Source: three-view drawing plus pictorial views. Frame: mm from the lowest corner of the part. A direction names the side the tool comes from. Coordinates: 2 decimals unless noted, no trailing zeros. Order: outer loops, then holes, each group sorted by start corner. A loop starts at its lowest first (then second) coordinate and runs counter-clockwise, first axis right, second up. Notation, with made-up numbers: (64.5, -17.75) -> (78.5, -17.75) arc R23 cw to (78.5, 19.25) -> close; hole circle Ø11 at (29.25, -32). An arc over 180 degrees is marked (long way). One line per question, with ' | ' between items.
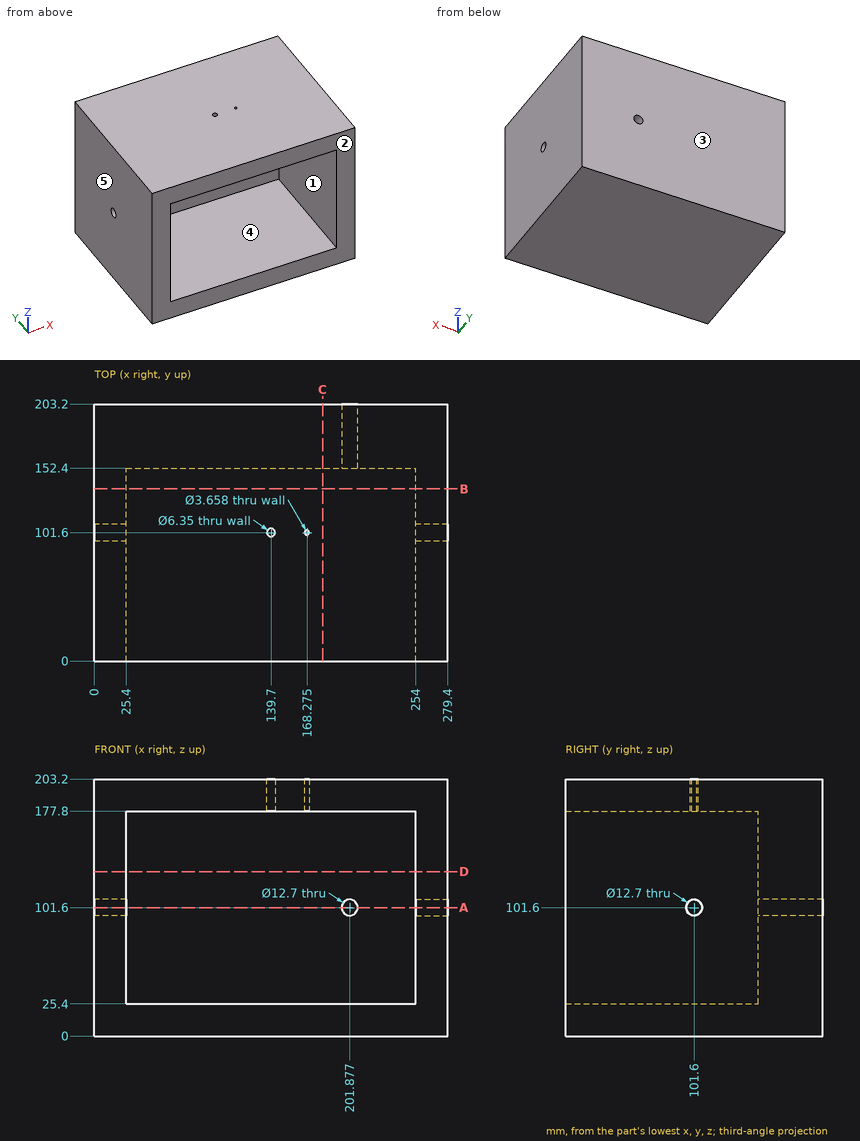
1. Mould query, pull axis X, two halves, no side actions, for the marked faces 3, 4 and 5. Classes: released by +X, released by -X, zero draft, split by the parting line, or undercut.
Recorded:
face 3: zero draft | face 4: undercut | face 5: released by -X
2. Cut plane D-D, the plane z = 130. Return loops of the section in (x, y), and give its area (3 significant figures).
Recorded:
outline: (0, 0) -> (25.4, 0) -> (25.4, 152.4) -> (254, 152.4) -> (254, 0) -> (279.4, 0) -> (279.4, 203.2) -> (0, 203.2) -> close | area: 21,900 mm^2
3. Ray query, line 1 (Z direction, x = 273, y = 101); line 2 (Z direction, x = 197.5, y = 103.5); line 3 (X direction, y = 72, z = 63). Return the intervals inside material, ascending. Write a range as [from, to].
Recorded:
line 1: z = [0, 95.28], [107.92, 203.2] | line 2: z = [0, 25.4], [177.8, 203.2] | line 3: x = [0, 25.4], [254, 279.4]
4. Cut plane A-A, the plane z = 101.6. Return loops of the section in (x, y), and give its area (3 significant figures).
Recorded:
outline: (0, 0) -> (25.4, 0) -> (25.4, 95.25) -> (0, 95.25) -> close; (0, 107.95) -> (25.4, 107.95) -> (25.4, 152.4) -> (195.53, 152.4) -> (195.53, 203.2) -> (0, 203.2) -> close; (208.23, 152.4) -> (254, 152.4) -> (254, 107.95) -> (279.4, 107.95) -> (279.4, 203.2) -> (208.23, 203.2) -> close; (254, 0) -> (279.4, 0) -> (279.4, 95.25) -> (254, 95.25) -> close | area: 20,600 mm^2
5. Pin query (flat end, axial travel): pin 1 Ø6 at (x, z) = (37.5, 169) entering from -Y. Return the tip coordinate at first contact, or that it passes through.
Recorded:
pin 1: stops at y = 152.4
6. Cut plane B-B, the plane y = 136. Return loops of the section in (x, z).
Recorded:
outline: (0, 0) -> (279.4, 0) -> (279.4, 203.2) -> (0, 203.2) -> close; hole (25.4, 25.4) -> (254, 25.4) -> (254, 177.8) -> (25.4, 177.8) -> close
7. Cut plane C-C, the plane x = 180.5. Return loops of the section in (y, z), and give its area (3 significant figures).
Recorded:
outline: (0, 0) -> (203.2, 0) -> (203.2, 203.2) -> (0, 203.2) -> (0, 177.8) -> (152.4, 177.8) -> (152.4, 25.4) -> (0, 25.4) -> close | area: 18,100 mm^2
8. Access query for the marked faces 1 and 2. Directions: +Z, -Z, +X, -X, +Y, -Y. A direction counts if a zero-diameter tool reaches every point of the face in a straight line with its end or side. Return the directions, or none.
Recorded:
face 1: -Y | face 2: +Z, -Z, +X, -X, -Y
